```python
from build123d import *

# Parameters (mm, degrees)
CUT_EXTRUDE1_DEPTH = 19.05


with BuildPart() as part:
    # Sketch1 → Revolve1 (revolve)
    with BuildSketch(Plane.XY, mode=Mode.PRIVATE) as revolve1_sk:
        Polygon((0, 0), (-8.255, 0), (-9.906, 2.54), (-9.144, 2.54), (-9.144, 6.35), (-10.795, 6.604), (-10.795, 11.43), (0, 11.43), align=None)
    revolve(revolve1_sk.sketch.rotate(Axis((0, 11.43, 0), (0, -1, 0)), 270), axis=Axis((0, 11.43, 0), (0, -1, 0)))  # turned: the seam where the file's is

    # Sketch2 → Cut-Extrude1 (cut, symmetric)
    with BuildSketch(Plane.XY):
        Polygon((7.14375, 6.298580206), (-7.14375, 6.298580206), (-7.14375, 8.863980206), (-5.08, 8.863980206), (-5.08, 11.43), (5.08, 11.43), (5.08, 8.863980206), (7.14375, 8.863980206), align=None)
    extrude(amount=CUT_EXTRUDE1_DEPTH, both=True, mode=Mode.SUBTRACT)


solid = part.part
```
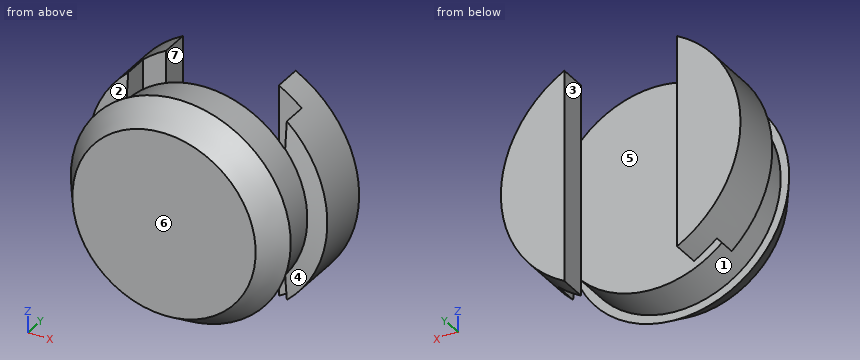
Work out the finished part from the listing and answer in its coordinate system (mm). Face numbers are marked on the shaded views. A direction names the side the tool comes from. Give positions to 0.01 mm unless a question says otherwise; leave off trailing zeros. Loops run counter-clockwise (first coordinate to the right, second up) from the corner with the lowest first, then second, coordinate; pieces in that order, holes last. Notation, with made-up numbers: (87, 45) - (124, 45) arc R21 cw to (124, 56) - close; hole circle Ø8 at (-19, 10). An arc over 180 degrees is marked (long way). One line per question, with ' | ' between items.
(1) The part is cut by section B-B (y = 8.5). Write down the section's boundary in (x, z) (3 decimals).
Recorded:
outline: (-7.144, -8.093) - (-7.144, 8.093) arc R10.795 ccw to start; (7.144, -8.093) arc R10.795 ccw to (7.144, 8.093) - close
(2) Each of these flat-tipped pins is pushed along its axis until it touches: pin 1 Ø3 at (x, y) = (6.5, 7) entering from +Z; pin 2 Ø3 at (y, z) = (7, 3.5) entering from -X; pin 3 Ø1.3 at (y, z) = (10.5, 3) entering from +X. Where does it stop, or does it pass through?
Recorded:
pin 1: stops at z = 8.09 | pin 2: stops at x = -10.61 | pin 3: stops at x = 10.54
(3) The part is cut by section A-A (z = 0). Write down the section's boundary in (x, y) (3 decimals), then the cut area to 3 significant figures.
Recorded:
outline: (-10.795, 6.604) - (-9.144, 6.35) - (-9.144, 2.54) - (-9.906, 2.54) - (-8.255, 0) - (8.255, 0) - (9.906, 2.54) - (9.144, 2.54) - (9.144, 6.35) - (10.795, 6.604) - (10.795, 11.43) - (5.08, 11.43) - (5.08, 8.864) - (7.144, 8.864) - (7.144, 6.299) - (-7.144, 6.299) - (-7.144, 8.864) - (-5.08, 8.864) - (-5.08, 11.43) - (-10.795, 11.43) - close | area: 162 mm²
(4) A tool of negligible diameter and unlimited length cuts with its end or side. For the marked faces 4, 5, 6 and 7, from which of +Z, -Z, +X, -X, +Y, -Y can it reach the whole face along a straight path? Write none if from no direction.
Recorded:
face 4: +X | face 5: +Z, -Z | face 6: +Z, -Z, +X, -X, -Y | face 7: +Z, -Z, +Y
(5) The mould has two halves that part along X. Classify the marked faces 1, 2 and 3: +X half, -X half, draft (parallel to the pull), parting line (faces both ways), or undercut.
Recorded:
face 1: parting line | face 2: -X half | face 3: undercut
(6) The part is cut by section C-C (x = 0). Write down the section's boundary in (y, z) (3 decimals).
Recorded:
outline: (0, -8.255) - (2.54, -9.906) - (2.54, -9.144) - (6.299, -9.144) - (6.299, 9.144) - (2.54, 9.144) - (2.54, 9.906) - (0, 8.255) - close
(7) Straight lines are drawn through the part: probe 1 along Y at (x, z) = (6.5, 1.75); probe 2 along X at (y, z) = (8.75, 0.25); probe 3 along Y at (x, z) = (1, 4.75). For each, find the intervals that lie inside material, in ascending order.
Recorded:
probe 1: y = 0 to 6.3, 8.86 to 11.43 | probe 2: x = -10.79 to -7.14, 7.14 to 10.79 | probe 3: y = 0 to 6.3
(8) The part is cut by section D-D (y = 9.75). Write down the section's boundary in (x, z) (3 decimals), then the cut area to 3 significant figures.
Recorded:
outline: (-5.08, -9.525) - (-5.08, 9.525) arc R10.795 ccw to start; (5.08, -9.525) arc R10.795 ccw to (5.08, 9.525) - close | area: 155 mm²
